Here's how the part is built. I have some questions about the finished solid (model axes, mm). A direction names the side the tool comes from. Coordinates: 2 decimals unless noted, no trailing zeros. Loops run counter-clockwise (first coordinate to the right, second up) from the corner with the lowest first, then second, coordinate; pieces in that order, holes last. Notation, with made-up numbers: (18.25, 52) -> (70.25, 52) arc R24 ccw to (70.25, 80) -> close; hole circle Ø4 at (41.25, 6). An arc over 180 degrees is marked (long way). Answer as a JSON object with one key per item and string values. Group by question number.
Q1. Thinking about a two-plate mould opening in X: for faces 3 (the flat face through (1219.2, -163, 464)), 4 (the flat face through (941, -276.225, 611)), 5 (the flat face through (601, 0, 451)), which applies, released by +X, released by -X, zero draft, split by the parting line, or undercut?
Q2. I want a section at A-A on z = 301. Write out the boundary of the cut face in (x, y) (3 decimals).
Q3. On a 3-axis mill with a long thin cutter (end or side, diameter ignored), from which of +Z, -Z, +X, -X, +Y, -Y can I reach the whole of each face in a straight line? I mean faces 1 (the flat face through (601, -155, 914.4)), 2 (the flat face through (939, -279.4, 426)). Say none if no direction works.
Q4. I want a section at C-C on x = 635.5. Write out the boundary of the cut face in (y, z), then the cut area to 3 significant figures.
Q5. I want a section at B-B on x = 916. Write out the boundary of the cut face in (y, z) (3 decimals).
Q6. I need wall thicknesses on line 1 (Y direction, x = 421, z = 399); line 2 (Z direction, x = 858, y = -309.5). Which ranges of each line are inside material? Lowest first, please.
Q7. I'm going to push flat-ended pins straight in: pin 1 (6 mm diameter, centred on x = 948, y = -284, fed in from -Z); pin 2 (10 mm diameter, centred on y = -58, z = 585, fed in from -X); pin 3 (1.9 mm diameter, centred on x = 664.5, z = 370.5, fed in from -Y) (3 decimals). Where does each tip first touch, or does it pass through?
```python
from build123d import *

# Parameters (mm, degrees)
F0_W     = 1219.2
F0_H     = 279.4
F1_DEPTH = 914.4
F3_DEPTH = 1219.2
F4_W     = 6.35
F4_H     = 863.6
F4_W_2   = 254
F4_H_2   = 203.2
F5_DEPTH = 3.175


with BuildPart() as f1:
    # F0 (on Top) → F1 (new body)
    with BuildSketch(Plane.XY):
        with Locations((609.6, -139.7)):
            Rectangle(F0_W, F0_H)
    extrude(amount=F1_DEPTH)

    # F2 (on face) → F3 (join, through all)
    with BuildSketch(Plane(origin=(0, 0, 0), x_dir=(0, -1, 0), z_dir=(-1, 0, 0))):
        with BuildLine():
            Line((304.8, 914.4), (279.4, 914.4))
            Line((279.4, 914.4), (279.4, 863.6))
            Line((279.4, 863.6), (304.8, 863.6))
            ThreePointArc((304.8, 863.6), (330.2, 889), (304.8, 914.4))
        make_face()
    extrude(amount=-F3_DEPTH)

    # F4 (on face) → F5 (cut)
    with BuildSketch(Plane.XZ.offset(279.4)):
        with Locations((663.575, 431.8)):
            Rectangle(F4_W, F4_H)
        with Locations((942.975, 609.6)):
            Rectangle(F4_W_2, F4_H_2)
    extrude(amount=-F5_DEPTH, mode=Mode.SUBTRACT)


solid = f1.part
```
Result set:
{
 "1": {"face 3": "released by +X", "face 4": "undercut", "face 5": "zero draft"},
 "2": {"outline": "(0, -279.4) -> (660.4, -279.4) -> (660.4, -276.225) -> (666.75, -276.225) -> (666.75, -279.4) -> (1219.2, -279.4) -> (1219.2, 0) -> (0, 0) -> close"},
 "3": {"face 1": "+Z, +X, -X, +Y, -Y", "face 2": "-Z, +X, -X, -Y"},
 "4": {"outline": "(-304.8, 863.6) -> (-279.4, 863.6) -> (-279.4, 0) -> (0, 0) -> (0, 914.4) -> (-304.8, 914.4) arc R25.4 ccw to start", "area": "258,000 mm²"},
 "5": {"outline": "(-304.8, 863.6) -> (-279.4, 863.6) -> (-279.4, 711.2) -> (-276.225, 711.2) -> (-276.225, 508) -> (-279.4, 508) -> (-279.4, 0) -> (0, 0) -> (0, 914.4) -> (-304.8, 914.4) arc R25.4 ccw to start"},
 "6": {"line 1": "y = -279.4 to 0", "line 2": "z = 864.04 to 913.96"},
 "7": {"pin 1": "stops at z = 863.6", "pin 2": "stops at x = 0", "pin 3": "stops at y = -276.225"}
}
